The listing builds one solid part. Answer for the finished solid, in the listing's coordinates (mm). A direction names the side the tool comes from. Round coordinates to 2 decimals unless told otherwise and drop trailing zeros. Order: outer loops, then holes, each group sorted by start corner. A loop starts at its lowest first (then second) coordinate and runs counter-clockwise, first axis right, second up. Notation, with made-up numbers: M -11.5,18 L 4.5,18 A19 cw 4.5,42 Z; hole C -38,-7.5 d6. An arc over 180 degrees is marked long. Write item = value, one per line. Start each with the question number.
(1) A cutting plane is placed at B-B, the plane x = 24.55. Determine the outline of the cut face in (y, z).
(2) This flat-tipped pin is pushed along its axis until it touches: pin 1 (3 mm diameter, centred on x = -24.55, y = -63.35, fed in from +Z). Where does it stop, or does it pass through?
(3) For a pull along Y with two mould halves and no side action, classify faces 3 (the face through (1, -41, 4)), 4 (the face through (-37.5, -58, 4)), 5 (the face through (-20.25, -59, 4)) as released by +Y, released by -Y, zero draft, split by the parting line, or undercut.
(4) A cutting plane is placed at D-D, the plane z = 2. Determine the outline of the cut face in (x, y), and give its area (3 significant figures).
(5) Which of the six approach directions +Z, -Z, +X, -X, +Y, -Y give full straight-line access (tool end or side, diameter ignored) to faces 1 (the face through (37.5, -59, 4)), 2 (the face through (0, -48.5, 4))?
(6) Straight lines are drawn through the part: probe 1 along Y at (x, z) = (1.5, 1.25); probe 2 along Y at (x, z) = (-24.55, 4.5); probe 3 along X at (y, z) = (-62.5, 0.5). For each, find the intervals that lie inside material, in ascending order. Write a range as from..to.
(7) A cutting plane is placed at C-C, the plane y = -53.65. Determine the outline of the cut face in (x, z).
(8) A cutting plane is placed at A-A, the plane y = -67.5. Determine the outline of the cut face in (x, z).
from build123d import *

# Parameters (mm, degrees)
SKETCH2_W           = 104
SKETCH2_H           = 66
BOSS_EXTRUDE1_DEPTH = 8
BOSS_EXTRUDE2_DEPTH = 8
SKETCH4_W           = 104
SKETCH4_H           = 10
CUT_EXTRUDE1_DEPTH  = 8
BOSS_EXTRUDE4_DEPTH = 8
CUT_EXTRUDE2_DEPTH  = 8
SKETCH9_R           = 2.5
CUT_EXTRUDE3_DEPTH  = 9
CUT_EXTRUDE4_REACH  = 10
SKETCH10_R          = 2.35
SKETCH10_W          = 40.5
SKETCH10_H          = 20
CUT_EXTRUDE5_REACH  = 10
SKETCH11_W          = 128
SKETCH11_H          = 82


with BuildPart() as part:
    # Sketch2 → Boss-Extrude1 (new body)
    with BuildSketch(Plane.XY):
        Rectangle(SKETCH2_W, SKETCH2_H)
    extrude(amount=BOSS_EXTRUDE1_DEPTH)

    # Sketch3 → Boss-Extrude2 (add, through all)
    with BuildSketch(Plane.XY.offset(8)):
        Polygon((-52, -17), (-60, -17), (-60, -22), (-64, -22), (-64, -2), (-60, -2), (-60, -7), (-52, -7), align=None)
        Polygon((-52, 13), (-60, 13), (-60, 8), (-64, 8), (-64, 28), (-60, 28), (-60, 23), (-52, 23), align=None)
        Polygon((52, -7), (52, -17), (60, -17), (60, -22), (64, -22), (64, -2), (60, -2), (60, -7), align=None)
        Polygon((-32.5, -33), (-32.5, -41), (-37.5, -41), (-37.5, -76), (37.5, -76), (37.5, -41), (32.5, -41), (32.5, -33), (17.5, -33), (17.5, -41), (-17.5, -41), (-17.5, -33), align=None)
    extrude(amount=-BOSS_EXTRUDE2_DEPTH)

    # Sketch4 → Cut-Extrude1 (cut)
    with BuildSketch(Plane.XY.offset(8)):
        with Locations((0, 28)):
            Rectangle(SKETCH4_W, SKETCH4_H)
    extrude(amount=-CUT_EXTRUDE1_DEPTH, mode=Mode.SUBTRACT)

    # Sketch6 → Boss-Extrude4 (add)
    with BuildSketch(Plane.XY.offset(8)):
        with BuildLine():
            Line((52, 17), (52, 0))
            Line((52, 0), (0, 0))
            Line((0, 0), (0, 23))
            Line((0, 23), (42, 23))
            ThreePointArc((42, 23), (57.458350242, 37.430583736), (52, 17))
        make_face()
    extrude(amount=-BOSS_EXTRUDE4_DEPTH)

    # Sketch8 → Cut-Extrude2 (cut)
    with BuildSketch(Plane.XY.offset(8)):
        with BuildLine():
            Line((47.287664075, 17.965775092), (41.287664075, 7.573470247))
            ThreePointArc((41.287664075, 7.573470247), (46.489081435, 5.649562257), (52, 5.028320703))
            Line((52, 5.028320703), (52, 17))
            ThreePointArc((52, 17), (49.590394027, 17.222145828), (47.287664075, 17.965775092))
        make_face()
    extrude(amount=-CUT_EXTRUDE2_DEPTH, mode=Mode.SUBTRACT)

    # Sketch9 → Cut-Extrude3 (cut, through all)
    with BuildSketch(Plane.XY.offset(8)):
        with Locations((51.798896932, 27.998161553)):
            Circle(SKETCH9_R)
    extrude(amount=-CUT_EXTRUDE3_DEPTH, mode=Mode.SUBTRACT)

    # Sketch10 → Cut-Extrude4 (cut, up to next)
    with BuildSketch(Plane.XY.offset(8), mode=Mode.PRIVATE) as cut_extrude4_sk1:
        with Locations((-24.55, -53.65)):
            Circle(SKETCH10_R)
    cut_extrude4_tool1 = extrude(cut_extrude4_sk1.sketch, amount=-CUT_EXTRUDE4_REACH, mode=Mode.PRIVATE) & part.part
    add(cut_extrude4_tool1.solids().sort_by_distance((-24.55, -53.65, 8))[0], mode=Mode.SUBTRACT)
    # Sketch10 → Cut-Extrude4 (cut, up to next)
    with BuildSketch(Plane.XY.offset(8), mode=Mode.PRIVATE) as cut_extrude4_sk2:
        with Locations((-24.55, -63.35)):
            Circle(SKETCH10_R)
    cut_extrude4_tool2 = extrude(cut_extrude4_sk2.sketch, amount=-CUT_EXTRUDE4_REACH, mode=Mode.PRIVATE) & part.part
    add(cut_extrude4_tool2.solids().sort_by_distance((-24.55, -63.35, 8))[0], mode=Mode.SUBTRACT)
    # Sketch10 → Cut-Extrude4 (cut, up to next)
    with BuildSketch(Plane.XY.offset(8), mode=Mode.PRIVATE) as cut_extrude4_sk3:
        with Locations((24.55, -63.35)):
            Circle(SKETCH10_R)
    cut_extrude4_tool3 = extrude(cut_extrude4_sk3.sketch, amount=-CUT_EXTRUDE4_REACH, mode=Mode.PRIVATE) & part.part
    add(cut_extrude4_tool3.solids().sort_by_distance((24.55, -63.35, 8))[0], mode=Mode.SUBTRACT)
    # Sketch10 → Cut-Extrude4 (cut, up to next)
    with BuildSketch(Plane.XY.offset(8), mode=Mode.PRIVATE) as cut_extrude4_sk4:
        with Locations((24.55, -53.65)):
            Circle(SKETCH10_R)
    cut_extrude4_tool4 = extrude(cut_extrude4_sk4.sketch, amount=-CUT_EXTRUDE4_REACH, mode=Mode.PRIVATE) & part.part
    add(cut_extrude4_tool4.solids().sort_by_distance((24.55, -53.65, 8))[0], mode=Mode.SUBTRACT)
    # Sketch10 → Cut-Extrude4 (cut, up to next)
    with BuildSketch(Plane.XY.offset(8), mode=Mode.PRIVATE) as cut_extrude4_sk5:
        with Locations((0, -58.5)):
            Rectangle(SKETCH10_W, SKETCH10_H)
    cut_extrude4_tool5 = extrude(cut_extrude4_sk5.sketch, amount=-CUT_EXTRUDE4_REACH, mode=Mode.PRIVATE) & part.part
    add(cut_extrude4_tool5.solids().sort_by_distance((0, -58.5, 8))[0], mode=Mode.SUBTRACT)

    # Sketch11 → Cut-Extrude5 (cut, up to next)
    with BuildSketch(Plane.XY.offset(8), mode=Mode.PRIVATE) as cut_extrude5_sk1:
        Rectangle(SKETCH11_W, SKETCH11_H)
    cut_extrude5_tool1 = extrude(cut_extrude5_sk1.sketch, amount=-CUT_EXTRUDE5_REACH, mode=Mode.PRIVATE) & part.part
    add(cut_extrude5_tool1.solids().sort_by_distance((0, 0, 8))[0], mode=Mode.SUBTRACT)


solid = part.part
Reported:
q1.outline = M -76,0 L -65.7,0 L -65.7,8 L -76,8 Z; M -61,0 L -56,0 L -56,8 L -61,8 Z; M -51.3,0 L -41,0 L -41,8 L -51.3,8 Z
q2.pin_1 = through
q3.face_3 = released by +Y
q3.face_4 = zero draft
q3.face_5 = undercut
q4.outline = M -37.5,-76 L 37.5,-76 L 37.5,-41 L -37.5,-41 Z; hole C -24.55,-63.35 d4.7; hole C -24.55,-53.65 d4.7; hole M -20.25,-68.5 L 20.25,-68.5 L 20.25,-48.5 L -20.25,-48.5 Z; hole C 24.55,-63.35 d4.7; hole C 24.55,-53.65 d4.7
q4.area = 1,750 mm²
q5.face_1 = +Z, -Z, +X, +Y, -Y
q5.face_2 = +Z, -Z
q6.probe_1 = -76..-68.5, -48.5..-41
q6.probe_2 = -76..-65.7, -61..-56, -51.3..-41
q6.probe_3 = -37.5..-26.74, -22.36..-20.25, 20.25..22.36, 26.74..37.5
q7.outline = M -37.5,0 L -26.9,0 L -26.9,8 L -37.5,8 Z; M -22.2,0 L -20.25,0 L -20.25,8 L -22.2,8 Z; M 20.25,0 L 22.2,0 L 22.2,8 L 20.25,8 Z; M 26.9,0 L 37.5,0 L 37.5,8 L 26.9,8 Z
q8.outline = M -37.5,0 L -20.25,0 L -20.25,8 L -37.5,8 Z; M 20.25,0 L 37.5,0 L 37.5,8 L 20.25,8 Z
